Check sheet for the modelled part. Datum: model origin and axes. Units: mm. A direction names the side the tool comes from. Round coordinates to 2 decimals unless told otherwise and drop trailing zeros. Write each loop counter-clockwise with the first axis right and the second up, starting at its lowest first coordinate (ties: lowest second). Pieces come first, ordered by that corner, then holes. Notation, with made-up numbers: M 45.5,-9.75 L 91.5,-9.75 A25 cw 91.5,4.25 Z; hole C 3,-3.75 d6. An arc over 180 degrees is marked long. One line per item, written item: value.
from build123d import *

# Parameters (mm, degrees)
SKETCH1_W               = 151
SKETCH1_H               = 90
BOSS_EXTRUDE1_DEPTH     = 3
SKETCH2_R               = 1.75
CUT_EXTRUDE1_DEPTH      = 176.812400018
FILLET1_R               = 2
SKETCH3_R               = 1.25
CUT_EXTRUDE2_DEPTH      = 176.812400018
CUT_EXTRUDE3_DEPTH      = 176.812400018
CUT_EXTRUDE3_DEPTH_BACK = 176.812400018
SKETCH4_W               = 25.1
SKETCH4_H               = 3.1


with BuildPart() as part:
    # Sketch1 → Boss-Extrude1 (new body)
    with BuildSketch(Plane(origin=(0, 0, 0), x_dir=(1, 0, 0), z_dir=(0, 1, 0))):
        with Locations((75.5, 45)):
            Rectangle(SKETCH1_W, SKETCH1_H)
    extrude(amount=BOSS_EXTRUDE1_DEPTH)

    # Sketch2 → Cut-Extrude1 (cut, through all)
    with BuildSketch(Plane(origin=(0, 3, 0), x_dir=(1, 0, 0), z_dir=(0, 1, 0))):
        with Locations(Location((146, 86, 0), (0, 0, 270))):
            Circle(SKETCH2_R)
        with Locations(Location((146, 4, 0), (0, 0, 270))):
            Circle(SKETCH2_R)
        with Locations(Location((6, 86, 0), (0, 0, 270))):
            Circle(SKETCH2_R)
        with Locations(Location((6, 4, 0), (0, 0, 270))):
            Circle(SKETCH2_R)
    extrude(amount=-CUT_EXTRUDE1_DEPTH, mode=Mode.SUBTRACT)

    # Fillet1
    fillet1_edges = [part.edges().sort_by_distance(p)[0] for p in [
        (0, 1.5, -90),
        (151, 1.5, -90),
        (151, 1.5, 0),
        (0, 1.5, 0),
    ]]
    fillet(fillet1_edges, radius=FILLET1_R)

    # Sketch3 → Cut-Extrude2 (cut, through all)
    with BuildSketch(Plane(origin=(0, 3, 0), x_dir=(1, 0, 0), z_dir=(0, 1, 0))):
        with Locations(Location((87, 75, 0), (0, 0, 270))):
            Circle(SKETCH3_R)
        with Locations(Location((29, 75, 0), (0, 0, 270))):
            Circle(SKETCH3_R)
        with Locations(Location((87, 25, 0), (0, 0, 270))):
            Circle(SKETCH3_R)
        with Locations(Location((29, 25, 0), (0, 0, 270))):
            Circle(SKETCH3_R)
    extrude(amount=-CUT_EXTRUDE2_DEPTH, mode=Mode.SUBTRACT)

    # Sketch4 → Cut-Extrude3 (cut, two sides: drawn at the far end of the back side and taken through both)
    with BuildSketch(Plane(origin=(0, 3, 0), x_dir=(1, 0, 0), z_dir=(0, 1, 0)).offset(-CUT_EXTRUDE3_DEPTH_BACK)):
        with Locations((97.55, 4.55)):
            Rectangle(SKETCH4_W, SKETCH4_H)
        with Locations((128.45, 4.55)):
            Rectangle(SKETCH4_W, SKETCH4_H)
    extrude(amount=CUT_EXTRUDE3_DEPTH + CUT_EXTRUDE3_DEPTH_BACK, mode=Mode.SUBTRACT)


solid = part.part
Q1. Sectioned sample at B-B on y = 1.95. State how many separate pieces and enclosed holes the cut face has, and give its area (3 significant figures).
Completed:
separate pieces: 1
enclosed holes: 10
area: 13,400 mm^2
Q2. Scan lines: line 1 (X direction, y = 2.45, z = -86); line 2 (X direction, y = 2, z = -6); line 3 (Z direction, x = 123, y = 1.2). Record each from-to range of solid material in increasing order. Write a range as [from, to].
Completed:
line 1: [0, 4.25], [7.75, 144.25], [147.75, 151]
line 2: [0, 85], [110.1, 115.9], [141, 151]
line 3: [-90, -6.1], [-3, 0]
Q3. Access from +Z, -Z, +X, -X, +Y, -Y to the whole of each face (thin tool, end or side, straight path). Record for faces 5 (the flat face through (74, 3, -46)), 6 (the flat face through (97, 1, -6.1)).
Completed:
face 5: +Z, -Z, +X, -X, +Y
face 6: +Y, -Y
Q4. Sectioned sample at C-C on x = 146. Enter the section's corners in (y, z), and give its area (3 significant figures).
Completed:
outline: M 0,-90 L 3,-90 L 3,-87.75 L 0,-87.75 Z; M 0,-84.25 L 3,-84.25 L 3,-5.75 L 0,-5.75 Z; M 0,-2.25 L 3,-2.25 L 3,0 L 0,0 Z
area: 249 mm^2
Q5. Draft check along Z on faces 1 (the flat face through (74, 0, -46)), 2 (the cylindrical face through (147.18, 1.52, -5.29)), 3 (the flat face through (85, 1, -5)), 4 (the flat face through (74, 1, 0)). Enter one of: pulls with the +Z half, pulls with the -Z half, needs draft (parallel to the pull), parting line crosses it, or undercut.
Completed:
face 1: needs draft
face 2: undercut
face 3: undercut
face 4: pulls with the +Z half
Q6. Sectioned sample at A-A on x = 129. Enter the section's corners in (y, z), and give its area (3 significant figures).
Completed:
outline: M 0,-90 L 3,-90 L 3,-6.1 L 0,-6.1 Z; M 0,-3 L 3,-3 L 3,0 L 0,0 Z
area: 261 mm^2
